Work out the finished part from the listing and answer in its coordinate system (mm). Face numbers are marked on the shaded views. A direction names the side the tool comes from. Give positions to 0.01 mm unless a question says otherwise; leave off trailing zeros. Loops run counter-clockwise (first coordinate to the right, second up) from the corner with the lowest first, then second, coordinate; pieces in that order, holes last. Notation, with made-up numbers: (-32.5, 18.25) - (-16.5, 18.25) arc R38 ccw to (-16.5, 57.25) - close; hole circle Ø3 at (-1.5, -38.75). An arc over 180 degrees is marked (long way). Use CSV: the item, a comma, the result in double quotes.
from build123d import *

# Parameters (mm, degrees)
F0_R     = 11
F1_DEPTH = 5
F2_R     = 8.5
F3_DEPTH = 85
F4_SIZE  = 1
F5_SIZE  = 1


with BuildPart() as f1:
    # F0 (on Front) → F1 (new body)
    with BuildSketch(Plane.XZ):
        Circle(F0_R)
    extrude(amount=F1_DEPTH)

    # F2 (on face) → F3 (join)
    with BuildSketch(Plane.XZ.offset(5)):
        Circle(F2_R)
    extrude(amount=F3_DEPTH)

    # F4
    f4_edges = [f1.edges().sort_by_distance(p)[0] for p in [
        (-11, 0, 0),
    ]]
    chamfer(f4_edges, length=F4_SIZE)

    # F5
    f5_edges = [f1.edges().sort_by_distance(p)[0] for p in [
        (-8.5, -90, 0),
    ]]
    chamfer(f5_edges, length=F5_SIZE)


solid = f1.part
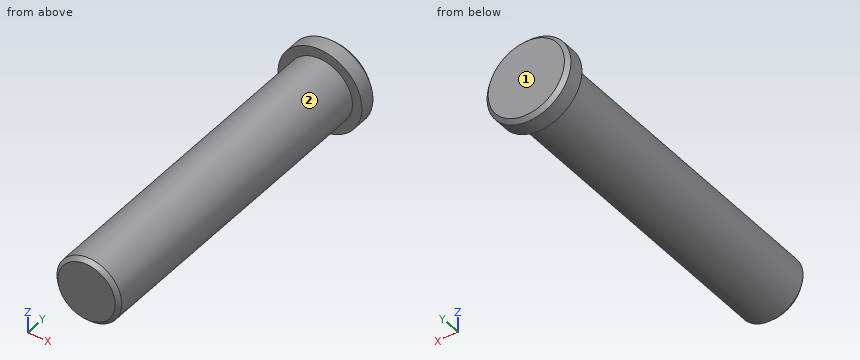
Item 1: For the marked faces 1 and 2, determine the directions among +Z, -Z, +X, -X, +Y, -Y from which every point of the face is accessible in a straight line to the end or side of a thin tool.
Determined:
face 1,"+Z, -Z, +X, -X, +Y"
face 2,"-Y"
Item 2: A cutting plane is placed at B-B on z = 0. Determine the outline of the cut face in (x, y), and give its area (3 significant figures).
Determined:
outline,"(-11, -5) - (-8.5, -5) - (-8.5, -89) - (-7.5, -90) - (7.5, -90) - (8.5, -89) - (8.5, -5) - (11, -5) - (11, -1) - (10, 0) - (-10, 0) - (-11, -1) - close"
area,"1,550 mm²"
Item 3: Given P1, Ø3, axis at x = -1.5, y = -27, coming from the +Z side; P2, Ø8, axis at y = -63.5, z = 0, coming from the +X side; P3, Ø5, axis at y = -79.5, z = -7, coming from the +X side, each flat-ended and moving along its own axis, determine where each tip first touches the part or whether it passes through.
Determined:
P1,"stops at z = 8.5"
P2,"stops at x = 8.5"
P3,"stops at x = 7.21"
Item 4: Find the intervals of material crossed by line 1 (Z direction, x = -6.5, y = -52.5); line 2 (Z direction, x = -3.75, y = -83.5); line 3 (Y direction, x = -8.5, z = -1), in increasing order.
Determined:
line 1,"z = -5.48 to 5.48"
line 2,"z = -7.63 to 7.63"
line 3,"y = -5 to 0"
Item 5: A cutting plane is placed at A-A on x = 0. Determine the outline of the cut face in (y, z), and give its area (3 significant figures).
Determined:
outline,"(-90, -7.5) - (-89, -8.5) - (-5, -8.5) - (-5, -11) - (-1, -11) - (0, -10) - (0, 10) - (-1, 11) - (-5, 11) - (-5, 8.5) - (-89, 8.5) - (-90, 7.5) - close"
area,"1,550 mm²"
Item 6: A cutting plane is placed at C-C on y = -10. Determine the outline of the cut face in (x, z), and give its area (3 significant figures).
Determined:
outline,"circle Ø17 at (0, 0)"
area,"227 mm²"
